Could you check a few things on this model? Use its own coordinates, in mm. A direction names the side the tool comes from. Coordinates: 2 decimals unless noted, no trailing zeros. Loops run counter-clockwise (first coordinate to the right, second up) from the corner with the lowest first, then second, coordinate; pieces in that order, holes last. Notation, with made-up numbers: (88, 72) - (129, 72) arc R20 ccw to (129, 100) - close; hole circle Ø10 at (-5, 1). An arc over 180 degrees is marked (long way). One line per question, with ' | ' between items. Start each with the question number.
1. I want a section at B-B, the plane x = 0. Write out the boundary of the cut face in (y, z).
2. We'd pull the mould along Y, two halves only. Please class faces 4 (the flat face through (0, 61, 9)), 5 (the flat face through (33.5, -22, 9)), 6 (the cylindrical face through (-30.49, 59.65, 9.42)): pulls with the +Y half, pulls with the -Y half, needs draft (parallel to the pull), parting line crosses it, or undercut.
3. Which directions (+Z, -Z, +X, -X, +Y, -Y) give clear straight access to the entire face, cutting with the end or side of a thin tool? Please do faces 1 (the cylindrical face through (29.58, 58.44, 9.44)), 2 (the conical face through (-29.09, 58.21, 13.91)), 3 (the flat face through (32.4, 9.5, 7.8)).
4. I want a section at A-A, the plane y = 40. Write out the boundary of the cut face in (x, z).
5. Please list where these lines run through material, in increasing order: L1, parallel to Y at x = -3, z = 8; L2, parallel to X at y = -29, z = 12.25; L3, parallel to Z at x = 24, y = -32. Write a range as [from, to].
6. I'm going to push flat-ended pins straight in: P1, Ø1.6, axis at x = 30.5, z = 10, coming from the -Y side; P2, Ø8, axis at x = 22.5, y = 0, coming from the +Z side; P3, Ø1.6, axis at y = 59.5, z = 6.5, coming from the +X side; P4, Ø7, axis at x = 0, y = 40, coming from the -Z side. Where does each tip first touch, or does it pass through?
from build123d import *

# Parameters (mm, degrees)
F1_DEPTH  = 15
F2_T      = -1.5
F3_R      = 6
F4_DEPTH  = 25
F5_R      = 4
F6_R      = 4
F12_DEPTH = 7
F13_W     = 7
F13_H     = 2.5
F14_DEPTH = 25


with BuildPart() as f1:
    # F0 (on Top) → F1 (new body)
    with BuildSketch(Plane.XY):
        with BuildLine():
            Line((23.5, 62.5), (-23.5, 62.5))
            ThreePointArc((-23.5, 62.5), (-30.5710678119, 59.5710678119), (-33.5, 52.5))
            Line((-33.5, 52.5), (-33.5, -52.5))
            ThreePointArc((-33.5, -52.5), (-30.5710678119, -59.5710678119), (-23.5, -62.5))
            Line((-23.5, -62.5), (23.5, -62.5))
            ThreePointArc((23.5, -62.5), (30.5710678119, -59.5710678119), (33.5, -52.5))
            Line((33.5, -52.5), (33.5, 52.5))
            ThreePointArc((33.5, 52.5), (30.5710678119, 59.5710678119), (23.5, 62.5))
        make_face()
    extrude(amount=F1_DEPTH)

    # F2
    f2_openings = [f1.faces().sort_by_distance(p)[0] for p in [
        (0, 0, 15),
    ]]
    offset(amount=F2_T, openings=f2_openings)

    # F3 (on face) → F4 (cut)
    with BuildSketch(Plane.XY.offset(1.5)):
        with Locations((0, 40)):
            Circle(F3_R)
    extrude(amount=-F4_DEPTH, mode=Mode.SUBTRACT)

    # F5
    f5_edges = [f1.edges().sort_by_distance(p)[0] for p in [
        (32, 0, 1.5),
        (29.510408, 58.510408, 1.5),
        (0, 61, 1.5),
        (-29.510408, 58.510408, 1.5),
        (-32, 0, 1.5),
        (-29.510408, -58.510408, 1.5),
        (0, -61, 1.5),
        (29.510408, -58.510408, 1.5),
    ]]
    fillet(f5_edges, radius=F5_R)

    # F6
    f6_edges = [f1.edges().sort_by_distance(p)[0] for p in [
        (-33.5, 0, 0),
        (-30.571068, 59.571068, 0),
        (-30.571068, -59.571068, 0),
        (0, -62.5, 0),
        (30.571068, -59.571068, 0),
        (33.5, 0, 0),
        (0, 62.5, 0),
        (30.571068, 59.571068, 0),
    ]]
    fillet(f6_edges, radius=F6_R)

    # F10: sweep along a path in F10_path
    with BuildLine(Plane(origin=(32, -52.5, 15), x_dir=(0, 1, 0), z_dir=(0, 0, 1))) as f10_path:
        Line((0, 0), (105, 0))
        ThreePointArc((105, 0), (111.0104076401, 2.4895923599), (113.5, 8.5))
        Line((113.5, 8.5), (113.5, 55.5))
        ThreePointArc((113.5, 55.5), (111.0104076401, 61.5104076401), (105, 64))
        Line((105, 64), (0, 64))
        ThreePointArc((0, 64), (-6.0104076401, 61.5104076401), (-8.5, 55.5))
        Line((-8.5, 55.5), (-8.5, 8.5))
    # F9 (on offset) → F10 (sweep)
    with BuildSketch(Plane.XZ.offset(52.5)):
        Polygon((32, 13.5), (32, 15), (31.3, 13.5), align=None)
    sweep(path=f10_path.line)

    # F11: sweep along a path in F11_path
    with BuildLine(Plane(origin=(23.5, -61, 15), x_dir=(0, -1, 0), z_dir=(0, 0, -1))) as f11_path:
        ThreePointArc((0, 0), (-2.4895923599, -6.0104076401), (-8.5, -8.5))
    # F9 (on offset) → F11 (sweep)
    with BuildSketch(Plane.XZ.offset(52.5)):
        Polygon((32, 13.5), (32, 15), (31.3, 13.5), align=None)
    sweep(path=f11_path.line)

    # F7 (on face) → F12 (cut)
    with BuildSketch(Plane.YZ.offset(33.5)):
        Polygon((25.5, 15), (9.5, 15), (9.5, 1.5), (25.5, 1.5), (25.5, 9.5), align=None)
    extrude(amount=-F12_DEPTH, mode=Mode.SUBTRACT)

    # F13 (on face) → F14 (cut)
    with BuildSketch(Plane(origin=(0, 62.5, 0), x_dir=(-1, 0, 0), z_dir=(0, 1, 0))):
        Polygon((-16, 10), (-16, 9.5), (-16, 4), (-9, 4), (-9, 10), align=None)
        with Locations((-12.5, 2.75)):
            Rectangle(F13_W, F13_H)
    extrude(amount=-F14_DEPTH, mode=Mode.SUBTRACT)


solid = f1.part
Results are:
1) outline: (-62.5, 4) arc R4 ccw to (-58.5, 0) - (34, 0) - (34, 1.5) - (-57, 1.5) arc R4 cw to (-61, 5.5) - (-61, 13.5) - (-60.3, 13.5) - (-61, 15) - (-62.5, 15) - close; (46, 0) - (58.5, 0) arc R4 ccw to (62.5, 4) - (62.5, 15) - (61, 15) - (60.3, 13.5) - (61, 13.5) - (61, 5.5) arc R4 cw to (57, 1.5) - (46, 1.5) - close
2) face 4: undercut | face 5: needs draft | face 6: pulls with the +Y half
3) face 1: none | face 2: +Z | face 3: +Z, +X
4) outline: (-33.5, 4) arc R4 ccw to (-29.5, 0) - (-6, 0) - (-6, 1.5) - (-28, 1.5) arc R4 cw to (-32, 5.5) - (-32, 13.5) - (-31.3, 13.5) - (-32, 15) - (-33.5, 15) - close; (6, 0) - (29.5, 0) arc R4 ccw to (33.5, 4) - (33.5, 15) - (32, 15) - (31.3, 13.5) - (32, 13.5) - (32, 5.5) arc R4 cw to (28, 1.5) - (6, 1.5) - close
5) L1: y = [-62.5, -61], [61, 62.5] | L2: x = [-33.5, -32], [32, 33.5] | L3: z = [0, 1.5]
6) P1: stops at y = -60.35 | P2: stops at z = 1.5 | P3: stops at x = 31.35 | P4: passes through
